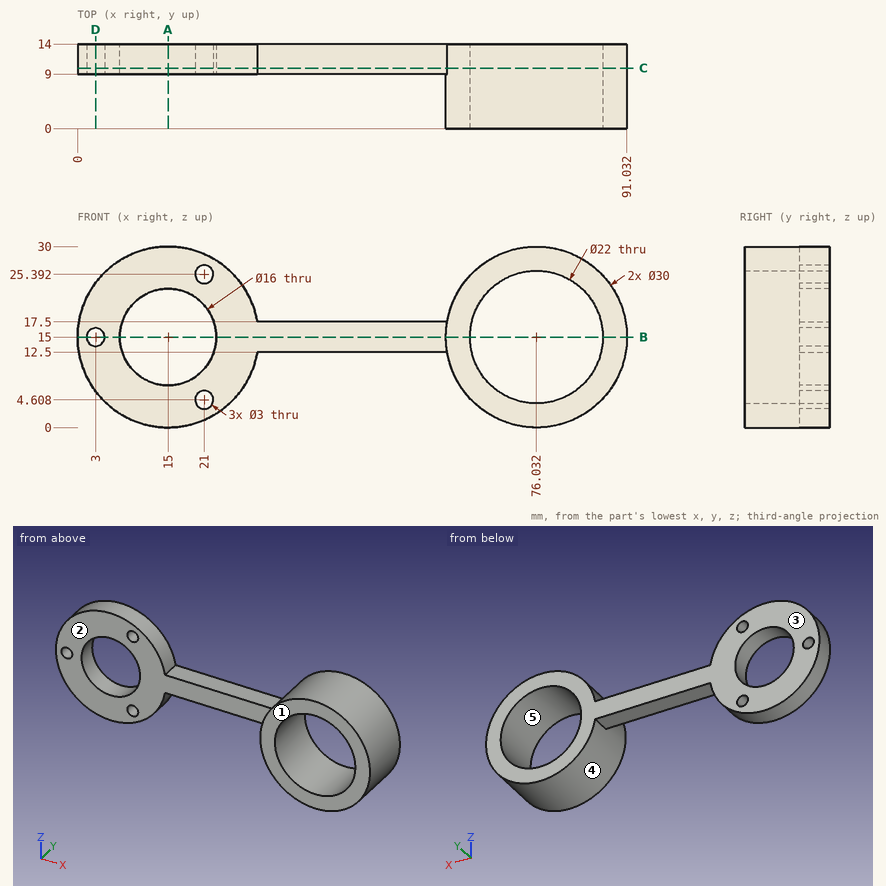
Could you check a few things on this drawing? It's one solid part, dimensions in mm from its lowest x, y, z. A direction names the side the tool comes from. Coordinates: 2 decimals unless noted, no trailing zeros. Write each loop counter-clockwise with the first axis right and the second up, starting at its lowest first coordinate (ties: lowest second). Pieces come first, ordered by that corner, then holes. Notation, with made-up numbers: (87.5, 31.25) - (124.5, 31.25) arc R23 cw to (124.5, 62.25) - close; hole circle Ø10 at (30.5, 46.5). An arc over 180 degrees is marked (long way). Put each result on its own line as item: value. Start each with the question number.
Q1. I want a section at B-B on z = 15. Write out the boundary of the cut face in (x, y), plus the area to 3 significant figures.
Q2. Which directions (+Z, -Z, +X, -X, +Y, -Y) give clear straight access to the entire face, cutting with the end or side of a thin tool? Please do the marked faces 1 and 2.
Q3. I'm going to push flat-ended pins straight in: P1, Ø6, axis at y = 3, z = 4, coming from the +X side; P2, Ø2, axis at x = 33.5, y = 11, coming from the +Z side; P3, Ø4, axis at x = 58.5, y = 9.5, coming from the -Z side; P4, Ø14.5, axis at x = 15, z = 15, coming from the -Y side. Where does each tip first touch, or does it pass through?
Q4. I want a section at D-D on x = 3. Write out the boundary of the cut face in (y, z).
Q5. I want a section at A-A on x = 15. Write out the boundary of the cut face in (y, z).
Q6. Thinking about a two-plate mould opening in Z: for the marked faces 3, 4 and 5, which applies, pulls with the +Z half, pulls with the -Z half, needs draft (parallel to the pull), parting line crosses it, or undercut?
Q7. I want a section at C-C on y = 10. Write out the boundary of the cut face in (x, z), plus the area to 3 significant figures.
Q8. Please list where these lines run through material, in increasing order: L1, parallel to Z at x = 15, y = 10.1; L2, parallel to Z at x = 21, y = 10.45; L3, parallel to X at y = 12, z = 3.5.
Checks:
1. outline: (0, 9) - (1.5, 9) - (1.5, 14) - (0, 14) - close; (4.5, 9) - (7, 9) - (7, 14) - (4.5, 14) - close; (23, 9) - (61.03, 9) - (61.03, 0) - (65.03, 0) - (65.03, 14) - (23, 14) - close; (87.03, 0) - (91.03, 0) - (91.03, 14) - (87.03, 14) - close
1. area: 322 mm²
2. face 1: +Z, -Z, +X, -X, -Y
2. face 2: +Z, -Z, -X, -Y
3. P1: x = 88.72
3. P2: z = 17.5
3. P3: z = 12.5
3. P4: through
4. outline: (9, 6) - (14, 6) - (14, 13.5) - (9, 13.5) - close; (9, 16.5) - (14, 16.5) - (14, 24) - (9, 24) - close
5. outline: (9, 0) - (14, 0) - (14, 7) - (9, 7) - close; (9, 23) - (14, 23) - (14, 30) - (9, 30) - close
6. face 3: needs draft
6. face 4: parting line crosses it
6. face 5: undercut
7. outline: (29.79, 12.5) - (61.24, 12.5) arc R15 ccw (long way) to (61.24, 17.5) - (29.79, 17.5) arc R15 ccw (long way) to start; hole circle Ø3 at (3, 15); hole circle Ø16 at (15, 15); hole circle Ø3 at (21, 4.61); hole circle Ø3 at (21, 25.39); hole circle Ø22 at (76.03, 15)
7. area: 967 mm²
8. L1: 0 to 7, 23 to 30
8. L2: 1.25 to 3.11, 6.11 to 9.71, 20.29 to 23.89, 26.89 to 28.75
8. L3: 5.37 to 19.99, 22.01 to 24.63, 66.4 to 85.66
